from build123d import *

# Parameters (mm, degrees)
CROQUIS1_W              = 33.552631578
CROQUIS1_H              = 30
SALIENTE_EXTRUIR1_DEPTH = 41.2
CROQUIS2_W              = 30
CROQUIS2_H              = 31.2
CORTAR_EXTRUIR1_DEPTH   = 36.2
CROQUIS3_R              = 2
CROQUIS3_R_2            = 1.25
CROQUIS3_R_3            = 3.71
CORTAR_EXTRUIR2_DEPTH   = 5
CROQUIS4_R              = 6
CORTAR_EXTRUIR3_DEPTH   = 5
REDONDEO1_R             = 2


with BuildPart() as part:
    # Croquis1 → Saliente-Extruir1 (new body)
    with BuildSketch(Plane(origin=(0, 0, 0), x_dir=(1, 0, 0), z_dir=(0, 1, 0))):
        Rectangle(CROQUIS1_W, CROQUIS1_H)
    extrude(amount=SALIENTE_EXTRUIR1_DEPTH)

    # Croquis2 → Cortar-Extruir1 (cut)
    with BuildSketch(Plane.XY.offset(15)):
        with Locations((-1.776315789, 20.6)):
            Rectangle(CROQUIS2_W, CROQUIS2_H)
    extrude(amount=-CORTAR_EXTRUIR1_DEPTH, mode=Mode.SUBTRACT)

    # Croquis3 → Cortar-Extruir2 (cut)
    with BuildSketch(Plane(origin=(0, 41.2, 0), x_dir=(1, 0, 0), z_dir=(0, 1, 0))):
        with Locations((-12.376315789, -12)):
            Circle(CROQUIS3_R)
        with Locations((-2.376315789, -11.563330836)):
            Circle(CROQUIS3_R_2)
        with Locations((7.623684211, -12)):
            Circle(CROQUIS3_R)
        with Locations((-2.376315789, -2)):
            Circle(CROQUIS3_R_3)
        with Locations((7.623684211, 8)):
            Circle(CROQUIS3_R)
        with Locations((-2.376315789, 8)):
            Circle(CROQUIS3_R_2)
        with Locations((-12.376315789, 8)):
            Circle(CROQUIS3_R)
    extrude(amount=-CORTAR_EXTRUIR2_DEPTH, mode=Mode.SUBTRACT)

    # Croquis4 → Cortar-Extruir3 (cut)
    with BuildSketch(Plane.XZ):
        with Locations((-2.779999999, 0)):
            Circle(CROQUIS4_R)
    extrude(amount=-CORTAR_EXTRUIR3_DEPTH, mode=Mode.SUBTRACT)

    # Redondeo1
    redondeo1_edges = [part.edges().sort_by_distance(p)[0] for p in [
        (-16.776315789, 36.2, 0),
    ]]
    fillet(redondeo1_edges, radius=REDONDEO1_R)


solid = part.part
Work out the finished part from the listing and answer in its coordinate system (mm). A direction names the side the tool comes from. Give positions to 0.01 mm unless a question says otherwise; leave off trailing zeros. Loops run counter-clockwise (first coordinate to the right, second up) from the corner with the lowest first, then second, coordinate; pieces in that order, holes last. Notation, with made-up numbers: (-39, 9) - (-9, 9) arc R19 cw to (-9, 19) - close; hole circle Ø3 at (84, 0). An arc over 180 degrees is marked (long way). Answer in a Markdown table with one row per item.
(1) For a pull along X with two mould halves and no side action, classify faces 4 (the face through (14, 22, -15)), 5 (the face through (-16.776, 40, 0)), 6 (the face through (2.943, 2.465, 1.802)) as pulls with the +X half, pulls with the -X half, needs draft (parallel to the pull), parting line crosses it, or undercut.
Results list:
| item | result |
|---|---|
| face 4 | needs draft |
| face 5 | pulls with the -X half |
| face 6 | undercut |
(2) A tool of negligible diameter and unlimited length cuts with its end or side. For faces 1 (the face through (0, 41.2, -4)), 2 (the face through (-2.647, 38.735, 12.784)), 3 (the face through (13.224, 20, 0)), from which of +Z, -Z, +X, -X, +Y, -Y can it reach the whole face along a straight path? Write none if from no direction.
Results list:
| item | result |
|---|---|
| face 1 | +Z, -Z, +X, -X, +Y |
| face 2 | +Y |
| face 3 | +Z, -Z, -X |
(3) Section D-D (z = -4) is taken. Give the vertices of the cut face in (x, y), and give its area (3 significant figures).
Results list:
| item | result |
|---|---|
| outline | (-16.78, 0) - (-7.25, 0) - (-7.25, 5) - (-16.78, 5) - close; (-16.78, 38.2) arc R2 ccw to (-14.78, 36.2) - (13.22, 36.2) - (13.22, 5) - (1.69, 5) - (1.69, 0) - (16.78, 0) - (16.78, 41.2) - (-16.78, 41.2) - close |
| area | 401 mm² |
(4) Section A-A (z = -8) is taken. Give the vertices of the cut face in (x, y), and give its area (3 significant figures).
Results list:
| item | result |
|---|---|
| outline | (-16.78, 0) - (16.78, 0) - (16.78, 41.2) - (9.62, 41.2) - (9.62, 36.2) - (13.22, 36.2) - (13.22, 5) - (-16.78, 5) - close; (-16.78, 38.2) arc R2 ccw to (-14.78, 36.2) - (-14.38, 36.2) - (-14.38, 41.2) - (-16.78, 41.2) - close; (-10.38, 36.2) - (-3.63, 36.2) - (-3.63, 41.2) - (-10.38, 41.2) - close; (-1.13, 36.2) - (5.62, 36.2) - (5.62, 41.2) - (-1.13, 41.2) - close |
| area | 393 mm² |
(5) Section C-C (x = -13) is taken. Give the vertices of the cut face in (y, z), and give its area (3 significant figures).
Results list:
| item | result |
|---|---|
| outline | (0, -15) - (5, -15) - (5, 15) - (0, 15) - close; (36.2, -15) - (41.2, -15) - (41.2, -9.9) - (36.2, -9.9) - close; (36.2, -6.1) - (41.2, -6.1) - (41.2, 10.1) - (36.2, 10.1) - close; (36.2, 13.9) - (41.2, 13.9) - (41.2, 15) - (36.2, 15) - close |
| area | 262 mm² |
(6) A flat-ended cylindrical pin translates along its axis: pin 1 Ø2 at (x, z) = (-2.38, -8) entering from +Y. Find the tip coordinate at first contact, or state that the pin passes through.
Results list:
| item | result |
|---|---|
| pin 1 | stops at y = 5 |
(7) Section B-B (x = -2.78) is taken. Give the vertices of the cut face in (y, z).
Results list:
| item | result |
|---|---|
| outline | (0, -15) - (5, -15) - (5, -6) - (0, -6) - close; (0, 6) - (5, 6) - (5, 15) - (0, 15) - close; (36.2, -15) - (41.2, -15) - (41.2, -9.18) - (36.2, -9.18) - close; (36.2, -6.82) - (41.2, -6.82) - (41.2, -1.69) - (36.2, -1.69) - close; (36.2, 5.69) - (41.2, 5.69) - (41.2, 10.38) - (36.2, 10.38) - close; (36.2, 12.75) - (41.2, 12.75) - (41.2, 15) - (36.2, 15) - close |
(8) Consider L1, parallel to Y at x = 6, z = -3.75; L2, parallel to X at y = 37.35, z = -8; L3, parallel to Y at x = 8, z = -9.75. Determine where each line is inside the solid, lowest interval first. Write a range as [from, to].
Results list:
| item | result |
|---|---|
| L1 | y = [0, 5], [36.2, 41.2] |
| L2 | x = [-16.59, -14.38], [-10.38, -3.63], [-1.13, 5.62], [9.62, 16.78] |
| L3 | y = [0, 5] |
